CAD build for the part. Positions are in the model's coordinates, mm. Round coordinates to 2 decimals unless told otherwise and drop trailing zeros. Order: outer loops, then holes, each group sorted by start corner. A loop starts at its lowest first (then second) coordinate and runs counter-clockwise, first axis right, second up. Notation, with made-up numbers: M 77,-27 L 92,-27 A17 ccw 92,2 Z; hole C 27.25,41 d9. An arc over 180 degrees is marked long. Put each result on its own line as item: value.
```python
from build123d import *

# Parameters (mm, degrees)
IZIM1_R                     = 2.65
IZIM1_R_2                   = 1.65
Y_KSEKLIK_EKSTR_ZYON1_DEPTH = 16
PAH1_SIZE                   = 0.1
IZIM2_R                     = 2.5
KES_EKSTR_ZYON1_DEPTH       = 8.8


with BuildPart() as part:
    # Çizim1 → Yükseklik-Ekstrüzyon1 (new body)
    with BuildSketch(Plane(origin=(0, 0, 0), x_dir=(1, 0, 0), z_dir=(0, 1, 0))):
        with Locations(Location((0, 0, 0), (0, 0, 270))):
            Circle(IZIM1_R)
        with Locations(Location((0, 0, 0), (0, 0, 270))):
            Circle(IZIM1_R_2, mode=Mode.SUBTRACT)
    extrude(amount=Y_KSEKLIK_EKSTR_ZYON1_DEPTH)

    # Pah1
    pah1_edges = [part.edges().sort_by_distance(p)[0] for p in [
        (0, 0, -2.65),
        (0, 16, -2.65),
    ]]
    chamfer(pah1_edges, length=PAH1_SIZE)

    # Çizim2 → Kes-Ekstrüzyon1 (cut, symmetric)
    with BuildSketch(Plane(origin=(0, 0, 0), x_dir=(0, 0, -1), z_dir=(1, 0, 0))):
        with Locations((4.25, 8)):
            Circle(IZIM2_R)
    extrude(amount=KES_EKSTR_ZYON1_DEPTH, both=True, mode=Mode.SUBTRACT)


solid = part.part
```
Item 1: Mould opens along Y. For faces 1 (the cylindrical face through (-1, 7.89, -1.31)), 2 (the cylindrical face through (0, 7.5, -1.8)), 3 (the flat face through (0, 0, 2)) say: pulls with the +Y half, pulls with the -Y half, needs draft (parallel to the pull), parting line crosses it, or undercut.
Answers below:
face 1: needs draft
face 2: undercut
face 3: pulls with the -Y half
Item 2: Band-saw the part on A-A on z = 0. Give the cut face in (x, y), and give its area (3 significant figures).
Answers below:
outline: M -2.65,0.1 L -2.55,0 L -1.65,0 L -1.65,16 L -2.55,16 L -2.65,15.9 Z; M 1.65,0 L 2.55,0 L 2.65,0.1 L 2.65,15.9 L 2.55,16 L 1.65,16 Z
area: 32.0 mm²
Item 3: Band-saw the part on D-D on y = 8.75. Give the cut face in (x, z).
Answers below:
outline: M -1.88,-1.87 L 1.88,-1.87 A2.65 ccw long Z; hole C 0,0 d3.3
Item 4: Band-saw the part on B-B on x = 0. Give the cut face in (y, z).
Answers below:
outline: M 0,-2.55 L 0.1,-2.65 L 6.08,-2.65 A2.5 cw 9.92,-2.65 L 15.9,-2.65 L 16,-2.55 L 16,-1.65 L 0,-1.65 Z; M 0,1.65 L 16,1.65 L 16,2.55 L 15.9,2.65 L 0.1,2.65 L 0,2.55 Z
Item 5: Band-saw the part on C-C on y = 13.25. Give the cut face in (x, z), and give its area (3 significant figures).
Answers below:
outline: C 0,0 d5.3; hole C 0,0 d3.3
area: 13.5 mm²
Item 6: Probe line 1 along X through (y, z) = (11, 0); line 2 along Z through (x, y) = (0.35, 1); line 3 along X through (y, z) = (1, -1.4). List the from-to ranges inside material, lowest first. Write a range as [from, to].
Answers below:
line 1: [-2.65, -1.65], [1.65, 2.65]
line 2: [-2.63, -1.61], [1.61, 2.63]
line 3: [-2.25, -0.87], [0.87, 2.25]
